The listing builds one solid part. Answer for the finished solid, in the listing's coordinates (mm). Round coordinates to 2 decimals unless told otherwise and drop trailing zeros. Write each loop counter-clockwise with the first axis right and the second up, starting at its lowest first coordinate (ties: lowest second). Pieces come first, ordered by that corner, then holes. Notation, with made-up numbers: (24, -29) - (38, -29) arc R34 ccw to (38, 4) - close; hole circle Ø5 at (-17, 63.25). An arc over 180 degrees is marked (long way). Answer in a Markdown table with one row per item.
Autodesk Inventor part; units mm, degrees
ref_plane "Startebene" through (0, 0, 0) normal (0, 0, 1) x (1, 0, 0)
ref_plane "Endebene" through (0, 0, 200) normal (0, 0, 1) x (1, 0, 0)
ref_plane "YZ Plane" through (0, 0, 0) normal (1, 0, 0) x (0, 1, 0)
ref_plane "Startebene" through (0, 0, 0) normal (0, 0, 1) x (1, 0, 0)
ref_plane "Endebene" through (0, 0, 200) normal (0, 0, 1) x (1, 0, 0)
sketch "Skizze" plane through (0, 0, 0) normal (0, 0, 1) x (1, 0, 0)
  line L0 (-10, -7) -> (-10, 7)
  line L1 (-7, 10) -> (7, 10)
  line L2 (10, 7) -> (10, -7)
  line L3 (7, -10) -> (-7, -10)
  arc A0 (-10, -7) -> (-7, -10) centre (-7, -7) ccw
  arc A1 (-7, 10) -> (-10, 7) centre (-7, 7) ccw
  arc A2 (10, 7) -> (7, 10) centre (7, 7) ccw
  arc A3 (7, -10) -> (10, -7) centre (7, -7) ccw
  arc A4 (-7, 8) -> (-8, 7) centre (-7, 7) ccw
  line L4 (-7, 8) -> (7, 8)
  arc A5 (8, 7) -> (7, 8) centre (7, 7) ccw
  line L5 (8, 7) -> (8, -7)
  arc A6 (7, -8) -> (8, -7) centre (7, -7) ccw
  line L6 (7, -8) -> (-7, -8)
  arc A7 (-8, -7) -> (-7, -8) centre (-7, -7) ccw
  line L7 (-8, -7) -> (-8, 7)
  line L8 (0, 37.1021) -> (0, -37.1021) construction
  line L9 (-23.1021, 0) -> (23.1021, 0) construction
  dimension "d7" = 3
  dimension "d10" = 20
  dimension "d11" = 20
  dimension "d12" = 2
  dimension "d15" = 10
  dimension "d16" = 10
extrude "Körper" add sketch "Skizze" along normal up to surface (200 mm away) from surface at 0
sketch "Sketch3" plane through (0, 0, 0) normal (0, 0, 1) x (1, 0, 0)
  line L0 (0, 0) -> (10, 0)
ref_plane "Work Plane3" through (0, 0, 0) normal (0, -1, 0) x (1, 0, 0)
sketch "Skizze5" plane through (10, -7, 200) normal (1, 0, 0) x (0, 0, -1)
  circle A0 centre (193.3333, 7) radius 0.9
  circle A1 centre (186.6667, 7) radius 0.9
  point P0 (200, 7)
hole "Bohrung1" at (10, 0, 6.6667) at (10, 0, 13.3333) direction (-1, 0, 0) diameter 2.3 depth 8 tip angle 118 countersink diameter 4.5 countersink angle 90
sketch "Skizze6" plane through (-10, 7, 0) normal (-1, 0, 0) x (0, 0, 1)
  circle A0 centre (6.6667, -7) radius 0.9
  circle A1 centre (13.3333, -7) radius 0.9
  point P0 (0, -7)
hole "Bohrung2" at (-10, 0, 6.6667) at (-10, 0, 13.3333) direction (1, 0, 0) diameter 2.3 depth 8 tip angle 118 countersink diameter 4.5 countersink angle 90
sketch "Skizze7" plane through (-7, -10, 0) normal (0, -1, 0) x (1, 0, 0)
  circle A0 centre (7, 6.6667) radius 0.9
  circle A1 centre (7, 13.3333) radius 0.9
  point P0 (7, 0)
hole "Bohrung3" at (0, -10, 6.6667) at (0, -10, 13.3333) direction (0, 1, 0) diameter 2.3 depth 8 tip angle 118 countersink diameter 4.5 countersink angle 90
sketch "Skizze8" plane through (7, 10, 200) normal (0, 1, 0) x (1, 0, 0)
  circle A0 centre (-7, 186.6667) radius 0.9
  circle A1 centre (-7, 193.3333) radius 0.9
  point P0 (-7, 200)
hole "Bohrung4" at (0, 10, 13.3333) at (0, 10, 6.6667) direction (0, -1, 0) diameter 2.3 depth 8 tip angle 118 countersink diameter 4.5 countersink angle 90
sketch "Skizze9" plane through (-7, -10, 0) normal (0, -1, 0) x (1, 0, 0)
  circle A0 centre (7, 140) radius 3
  line L0 (7, 140) -> (7, 200)
  line L1 (14, 200) -> (0, 200)
  line L2 (14, 200) -> (0, 200)
  point P0 (7, 0)
  dimension "d47" = 6
  dimension "d48" = 60
extrude "Extrusion2" cut sketch "Skizze9" against normal through all
sketch "Skizze10" plane through (10, -7, 200) normal (1, 0, 0) x (0, 0, -1)
  line L0 (200, 14) -> (0, 14) construction
  line L1 (100, 14) -> (100, 7) construction
  line L2 (100, 7) -> (100, 0) construction
  line L3 (200, 0) -> (0, 0) construction
  line L4 (57, 17) -> (63, 17) construction
  point P0 (200, 7)
  point P1 (60, 17)
  dimension "d51" = 40
hole "Bohrung5" at (10, 0, 100) direction (-1, 0, 0) diameter 2.459 end through all
sketch "Skizze11" plane through (-10, 7, 0) normal (-1, 0, 0) x (0, 0, 1)
  line L0 (196, -7) -> (200, -7)
  line L1 (200, -14) -> (200, 0)
  point P0 (0, -7)
  dimension "d59" = 4
hole "Bohrung6" at (-10, 0, 196) direction (1, 0, 0) diameter 3 end through all
sketch "Sketch4" plane through (0, 0, 0) normal (0, -1, 0) x (1, 0, 0)
  line L0 (-2, 0) -> (12, 0)
  line L1 (-2, 200) -> (12, 200)
  dimension "d18" = 200
equation "\"d7\" = G_IR"
equation "\"d10\" = G_H"
equation "\"d11\" = G_W"
equation "\"d12\" = G_T"
equation "\"d15\" = 0.5 * d10"
equation "\"d16\" = 0.5 * d11"
equation "\"d3\" = G_L"
equation "\"G_W\" = 20"
equation "\"G_H\" = 20"
equation "\"G_T\" = 2"
equation "\"G_IR\" = 3"
equation "\"G_L\" = d18"
equation "\"G_OFFSET_START\" = 0"
equation "\"G_OFFSET_END\" = 0"
properties part number "ISO 12633-2 - 20x20x2 - 200" material "Stahl, weich"
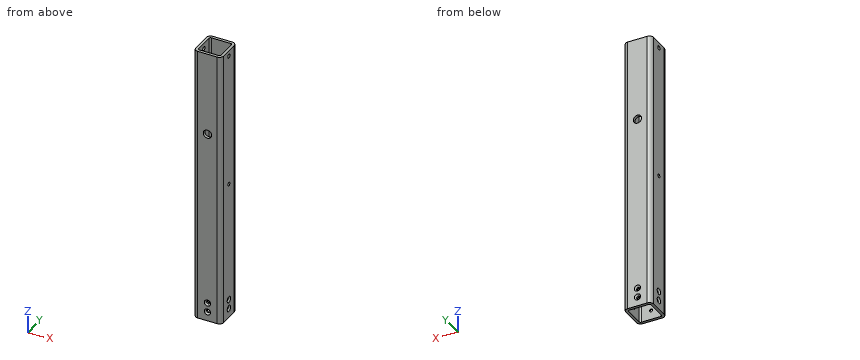
(1) Section C-C (z = 180.5) is taken. Give the vertices of the cut face in (x, y), and give its area (3 significant figures).
Checked values:
| item | result |
|---|---|
| outline | (-10, -7) arc R3 ccw to (-7, -10) - (7, -10) arc R3 ccw to (10, -7) - (10, 7) arc R3 ccw to (7, 10) - (-7, 10) arc R3 ccw to (-10, 7) - close; hole (-8, -7) arc R1 ccw to (-7, -8) - (7, -8) arc R1 ccw to (8, -7) - (8, 7) arc R1 ccw to (7, 8) - (-7, 8) arc R1 ccw to (-8, 7) - close |
| area | 137 mm2 |
(2) Section B-B (x = -5.25) is taken. Give the vertices of the cut face in (y, z).
Checked values:
| item | result |
|---|---|
| outline | (-10, 0) - (-8, 0) - (-8, 200) - (-10, 200) - close; (8, 0) - (10, 0) - (10, 200) - (8, 200) - close |
(3) Flat-ended cylindrical pins translate along their axes: pin 1 (2.5 mm diameter, centred on x = 0, z = 13.33, fed in from -Y); pin 2 (3.5 mm diameter, centred on x = 0, z = 6.67, fed in from +Y); pin 3 (3 mm diameter, centred on y = 0, z = 13.33, fed in from -X). Find the tip coordinate at first contact, or state that the pin passes through.
Checked values:
| item | result |
|---|---|
| pin 1 | stops at y = -9 |
| pin 2 | stops at y = 9.5 |
| pin 3 | stops at x = -9.25 |
(4) Section A-A (z = 140) is taken. Give the vertices of the cut face in (x, y), and give its area (3 significant figures).
Checked values:
| item | result |
|---|---|
| outline | (-10, -7) arc R3 ccw to (-7, -10) - (-3, -10) - (-3, -8) - (-7, -8) arc R1 cw to (-8, -7) - (-8, 7) arc R1 cw to (-7, 8) - (-3, 8) - (-3, 10) - (-7, 10) arc R3 ccw to (-10, 7) - close; (3, -10) - (7, -10) arc R3 ccw to (10, -7) - (10, 7) arc R3 ccw to (7, 10) - (3, 10) - (3, 8) - (7, 8) arc R1 cw to (8, 7) - (8, -7) arc R1 cw to (7, -8) - (3, -8) - close |
| area | 113 mm2 |
(5) Find the intervals of material crossed by line 1 (Z direction, x = 8.2, y = 0); line 2 (Z direction, x = 0, y = 8.8); line 3 (X direction, y = -2, z = 84), in increasing order.
Checked values:
| item | result |
|---|---|
| line 1 | z = 0 to 5.52, 7.82 to 12.18, 14.48 to 98.77, 101.23 to 194.5, 197.5 to 200 |
| line 2 | z = 0 to 5.52, 7.82 to 12.18, 14.48 to 137, 143 to 200 |
| line 3 | x = -10 to -8, 8 to 10 |
